Autodesk Inventor part; units mm, degrees
ref_plane "YZ Plane" through (0, 0, 0) normal (1, 0, 0) x (0, 1, 0)
ref_plane "XZ Plane" through (0, 0, 0) normal (0, 1, 0) x (-1, 0, 0)
ref_plane "XY Plane" through (0, 0, 0) normal (0, 0, 1) x (1, 0, 0)
sketch "Sketch1" plane through (0, 0, 0) normal (0, 0, 1) x (1, 0, 0)
  line L0 (0, 0) -> (41, 0) construction
  line L1 (41, 0) -> (41, 65.3) construction
  line L2 (41, 65.3) -> (0, 65.3) construction
  circle A0 centre (20.5, 32.65) radius 8.5
  line L3 (0, 0) -> (41, 0)
  line L4 (41, 65.3) -> (0, 65.3)
  line L5 (20.5, 65.3) -> (20.5, 0) construction
  line L6 (0, 32.65) -> (41, 32.65) construction
  line L7 (0, 65.3) -> (0, 46.9591) construction
  line L8 (0, 18.3409) -> (0, 0) construction
  line L9 (0, 65.3) -> (0, 46.9591)
  line L10 (0, 18.3409) -> (0, 0)
  line L11 (41, 0) -> (41, 18.3409)
  line L12 (41, 46.9591) -> (41, 65.3)
  arc A1 (0, 46.9591) -> (0, 18.3409) centre (20.5, 32.65) ccw
  arc A2 (41, 18.3409) -> (41, 46.9591) centre (20.5, 32.65) ccw
  point P0 (5, 60.3)
  point P1 (36, 60.3)
  point P2 (5, 5)
  point P3 (36, 5)
  point P4 (12, 41.15)
  point P5 (8, 45.15)
  point P6 (29, 41.15)
  point P7 (33, 45.15)
  point P8 (29, 24.15)
  point P9 (12, 24.15)
  point P10 (8, 20.15)
  point P11 (33, 20.15)
  dimension "d3" = 17
  dimension "d5" = 5
  dimension "d6" = 5
  dimension "d7" = 5
  dimension "d10" = 12.5
  dimension "d11" = 25
  dimension "d12" = 25
  dimension "d13" = 17
  dimension "d14" = 17
  dimension "d15" = 8.5
  dimension "d16" = 24.15
  dimension "d17" = 20.15
  dimension "d18" = 32.65
  dimension "d20" = 41
  dimension "d22" = 65.3
  dimension "d23" = 5
  dimension "d25" = 41
  dimension "d26" = 5
  dimension "d27" = 16.5
extrude "Extrusion1" add sketch "Sketch1" along normal blind 3
sketch "Sketch2" plane through (0, 0, 0) normal (0, 0, 1) x (1, 0, 0)
  line L0 (0, 0) -> (41, 0) construction
  line L1 (41, 0) -> (41, 65.3) construction
  line L2 (41, 65.3) -> (0, 65.3) construction
  circle A0 centre (20.5, 32.65) radius 8.5
  line L3 (0, 0) -> (41, 0)
  line L4 (41, 65.3) -> (0, 65.3)
  line L5 (20.5, 65.3) -> (20.5, 0) construction
  line L6 (0, 32.65) -> (41, 32.65) construction
  line L7 (0, 65.3) -> (0, 46.9591) construction
  line L8 (0, 18.3409) -> (0, 0) construction
  line L9 (0, 65.3) -> (0, 46.9591)
  line L10 (0, 18.3409) -> (0, 0)
  line L11 (41, 0) -> (41, 18.3409)
  line L12 (41, 46.9591) -> (41, 65.3)
  arc A1 (0, 46.9591) -> (0, 18.3409) centre (20.5, 32.65) ccw
  arc A2 (41, 18.3409) -> (41, 46.9591) centre (20.5, 32.65) ccw
  point P0 (5, 60.3)
  point P1 (36, 60.3)
  point P2 (5, 5)
  point P3 (36, 5)
  point P4 (12, 41.15)
  point P5 (8, 45.15)
  point P6 (29, 41.15)
  point P7 (33, 45.15)
  point P8 (29, 24.15)
  point P9 (12, 24.15)
  point P10 (8, 20.15)
  point P11 (33, 20.15)
  dimension "d30" = 17
  dimension "d31" = 5
  dimension "d32" = 5
  dimension "d33" = 5
  dimension "d34" = 12.5
  dimension "d35" = 25
  dimension "d36" = 25
  dimension "d37" = 17
  dimension "d38" = 17
  dimension "d39" = 8.5
  dimension "d40" = 24.15
  dimension "d41" = 20.15
  dimension "d42" = 32.65
  dimension "d43" = 41
  dimension "d44" = 65.3
  dimension "d45" = 5
  dimension "d46" = 41
  dimension "d47" = 5
  dimension "d48" = 16.5
hole "Hole1" at (5, 60.3, 0) at (36, 60.3, 0) at (5, 5, 0) at (36, 5, 0) at (12, 41.15, 0) at (8, 45.15, 0) at (29, 41.15, 0) at (33, 45.15, 0) at (29, 24.15, 0) at (12, 24.15, 0) at (8, 20.15, 0) at (33, 20.15, 0) direction (0, 0, 1) diameter 3.3 end through all
sketch "Sketch3" plane through (0, 0, 3) normal (0, 0, 1) x (1, 0, 0)
  circle A0 centre (8, 45.15) radius 1.65
  line L0 (9.1667, 46.3167) -> (13.1667, 42.3167)
  circle A1 centre (12, 41.15) radius 1.65
  circle A2 centre (33, 20.15) radius 1.65
  circle A3 centre (29, 24.15) radius 1.65
  circle A4 centre (33, 20.15) radius 1.65
  circle A5 centre (29, 24.15) radius 1.65
  line L1 (10.8333, 39.9833) -> (6.8333, 43.9833)
  circle A6 centre (33, 45.15) radius 1.65
  circle A7 centre (29, 41.15) radius 1.65
  circle A8 centre (33, 45.15) radius 1.65
  circle A9 centre (8, 20.15) radius 1.65
  line L2 (6.8333, 21.3167) -> (10.8333, 25.3167)
  line L3 (13.1667, 22.9833) -> (9.1667, 18.9833)
  circle A10 centre (12, 24.15) radius 1.65
  line L4 (27.8333, 42.3167) -> (31.8333, 46.3167)
  line L5 (30.1667, 39.9833) -> (34.1667, 43.9833)
  line L6 (27.8333, 22.9833) -> (31.8333, 18.9833)
  line L7 (34.1667, 21.3167) -> (30.1667, 25.3167)
  point P0 (0, 0)
extrude "Extrusion2" cut sketch "Sketch3" against normal blind 3 contours A0 L0 A1 L1 | A2 L6 A3 L7 | A6 L5 A7 L4 | A9 L2 A10 L3
fillet "Fillet1" radius 3 4 edges at (41, 65.3, 1.5) (0, 65.3, 1.5) (0, 0, 1.5) (41, 0, 1.5)
sketch "Sketch4" plane through (0, 0, 3) normal (0, 0, 1) x (1, 0, 0)
  line L0 (13.1667, 22.9833) -> (9.1667, 18.9833)
  arc A0 (6.8333, 21.3167) -> (9.1667, 18.9833) centre (8, 20.15) ccw
  line L1 (6.8333, 21.3167) -> (10.8333, 25.3167)
  arc A1 (13.1667, 22.9833) -> (10.8333, 25.3167) centre (12, 24.15) ccw
  line L2 (31.8333, 18.9833) -> (27.8333, 22.9833)
  arc A2 (30.1667, 25.3167) -> (27.8333, 22.9833) centre (29, 24.15) ccw
  line L3 (30.1667, 25.3167) -> (34.1667, 21.3167)
  arc A3 (31.8333, 18.9833) -> (34.1667, 21.3167) centre (33, 20.15) ccw
  line L4 (34.1667, 43.9833) -> (30.1667, 39.9833)
  arc A4 (27.8333, 42.3167) -> (30.1667, 39.9833) centre (29, 41.15) ccw
  line L5 (27.8333, 42.3167) -> (31.8333, 46.3167)
  arc A5 (34.1667, 43.9833) -> (31.8333, 46.3167) centre (33, 45.15) ccw
  circle A6 centre (5, 5) radius 1.65
  circle A7 centre (5, 60.3) radius 1.65
  circle A8 centre (36, 60.3) radius 1.65
  circle A9 centre (36, 5) radius 1.65
  line L6 (10.8333, 39.9833) -> (6.8333, 43.9833)
  arc A10 (9.1667, 46.3167) -> (6.8333, 43.9833) centre (8, 45.15) ccw
  line L7 (9.1667, 46.3167) -> (13.1667, 42.3167)
  arc A11 (10.8333, 39.9833) -> (13.1667, 42.3167) centre (12, 41.15) ccw
  circle A12 centre (20.5, 32.65) radius 8.5
  arc A13 (38, 0) -> (41, 3) centre (38, 3) ccw
  line L8 (41, 3) -> (41, 18.3409)
  arc A14 (41, 18.3409) -> (41, 46.9591) centre (20.5, 32.65) ccw
  line L9 (41, 46.9591) -> (41, 62.3)
  arc A15 (41, 62.3) -> (38, 65.3) centre (38, 62.3) ccw
  line L10 (38, 65.3) -> (3, 65.3)
  arc A16 (3, 65.3) -> (0, 62.3) centre (3, 62.3) ccw
  line L11 (0, 62.3) -> (0, 46.9591)
  arc A17 (0, 46.9591) -> (0, 18.3409) centre (20.5, 32.65) ccw
  line L12 (0, 18.3409) -> (0, 3)
  arc A18 (0, 3) -> (3, 0) centre (3, 3) ccw
  line L13 (3, 0) -> (38, 0)
  point P0 (0, 0)
properties part number "TapaSuperior"
Work out the finished part from the listing and answer in its coordinate system (mm). A direction names the side the tool comes from. Coordinates: 2 decimals unless noted, no trailing zeros. Write each loop counter-clockwise with the first axis right and the second up, starting at its lowest first coordinate (ties: lowest second). Pieces come first, ordered by that corner, then holes. Notation, with made-up numbers: M 32.25,11 L 61.25,11 A30 ccw 61.25,34 Z; hole C 36,80 d7. An arc over 180 degrees is marked long. Use one line per item in the form item = value. Start each with the question number.
1. The mould has two halves that part along Y. Classify faces 4 (the face through (34.61, 61.19, 1.52)), 5 (the face through (0, 55, 1)), 6 (the face through (13.141, 39.958, 1.521)), 7 (the face through (0.86, 0.9, 1.52)): released by +Y, released by -Y, zero draft, split by the parting line, or undercut.
2. Straight lines are drawn through the part: probe 1 along Y at (x, z) = (5, 1.6); probe 2 along X at (y, z) = (60.3, 1.25); probe 3 along Y at (x, z) = (34, 2.1). For each, find the intervals that lie inside material, in ascending order. Write a range as from..to.
3. Each of these flat-tipped pins is pushed along its axis until it touches: P1, Ø0.9, axis at y = 51.5, z = 1, coming from the +X side; P2, Ø1.5, axis at y = 57, z = 2, coming from the -X side; P3, Ø3, axis at x = 27.5, y = 52.5, coming from the -Z side. Where does it stop, or does it pass through?
4. A tool of negligible diameter and unlimited length cuts with its end or side. For faces 1 (the face through (20, 0, 1)), 2 (the face through (29.805, 21.011, 1.521)), 3 (the face through (41, 11, 1)), from which of +Z, -Z, +X, -X, +Y, -Y can it reach the whole face along a straight path? Write none if from no direction.
5. The part is cut by section B-B (x = 5). Give the vertices of the cut face in (y, z).
6. The part is cut by section D-D (x = 20.5). Give the vertices of the cut face in (y, z).
7. The part is cut by section C-C (y = 32.65). Give the vertices of the cut face in (x, z), plus the area to 3 significant figures.
8. The part is cut by section A-A (y = 5). Give the vertices of the cut face in (x, z).
Evaluation:
q1.face_4 = undercut
q1.face_5 = zero draft
q1.face_6 = undercut
q1.face_7 = released by -Y
q2.probe_1 = 0..3.35, 6.65..58.65, 61.95..65.3
q2.probe_2 = 0..3.35, 6.65..34.35, 37.65..41
q2.probe_3 = 0..18.84, 21.48..43.82, 46.46..65.3
q3.P1 = 41
q3.P2 = 0
q3.P3 = 0
q4.face_1 = +Z, -Z, +X, -X, -Y
q4.face_2 = +Z, -Z
q4.face_3 = +Z, -Z, +X, -Y
q5.outline = M 0,0 L 3.35,0 L 3.35,3 L 0,3 Z; M 6.65,0 L 58.65,0 L 58.65,3 L 6.65,3 Z; M 61.95,0 L 65.3,0 L 65.3,3 L 61.95,3 Z
q6.outline = M 0,0 L 24.15,0 L 24.15,3 L 0,3 Z; M 41.15,0 L 65.3,0 L 65.3,3 L 41.15,3 Z
q7.outline = M -4.5,0 L 12,0 L 12,3 L -4.5,3 Z; M 29,0 L 45.5,0 L 45.5,3 L 29,3 Z
q7.area = 99.0 mm^2
q8.outline = M 0,0 L 3.35,0 L 3.35,3 L 0,3 Z; M 6.65,0 L 34.35,0 L 34.35,3 L 6.65,3 Z; M 37.65,0 L 41,0 L 41,3 L 37.65,3 Z
